```python
from build123d import *

# Parameters (mm, degrees)
SKETCH1_R                = 4.25
EXTRUDE1_DEPTH           = 6
PROCESS_BENDS1_START     = -45.500357344
PROCESS_BENDS1_OUTLINE_W = 30
PROCESS_BENDS1_OUTLINE_H = 6
PROCESS_BENDS1_DEPTH     = 45.500357344
PROCESS_BENDS1_START_2   = -50.267477344
PROCESS_BENDS1_2_DEPTH   = 4.83288
PROCESS_BENDS1_START_3   = -56.267477344
PROCESS_BENDS1_3_DEPTH   = 6
PROCESS_BENDS1_START_4   = -45.434597344
PROCESS_BENDS1_4_DEPTH   = 1.16712
PROCESS_BENDS1_START_5   = -21
PROCESS_BENDS1_5_DEPTH   = 30


with BuildPart() as part:
    # Sketch1 → Extrude1 (new body)
    with BuildSketch(Plane.XY):
        with BuildLine():
            Line((-106.422252789, 9), (-40.637070261, 9))
            ThreePointArc((-40.637070261, 9), (-40.099770652, 8.843391446), (-39.730762474, 8.422618262))
            Line((-39.730762474, 8.422618262), (-38.495606339, 5.773817383))
            ThreePointArc((-38.495606339, 5.773817383), (-34.805524552, 1.566085542), (-29.432528469, 0))
            Line((-29.432528469, 0), (-3, 0))
            ThreePointArc((-3, 0), (-0.878679656, -0.878679656), (0, -3))
            Line((0, -3), (0, -7.904690938))
            ThreePointArc((0, -7.904690938), (-0.540498847, -9.622495956), (-1.967236053, -10.721319886))
            Line((-1.967236053, -10.721319886), (-29.49989713, -20.816628948))
            ThreePointArc((-29.49989713, -20.816628948), (-30.008202711, -20.95380152), (-30.532661077, -21))
            Line((-30.532661077, -21), (-159, -21))
            ThreePointArc((-159, -21), (-161.121320344, -20.121320344), (-162, -18))
            Line((-162, -18), (-162, 12))
            ThreePointArc((-162, 12), (-161.121320344, 14.121320344), (-159, 15))
            Line((-159, 15), (-122.577747211, 15))
            ThreePointArc((-122.577747211, 15), (-122.010424647, 14.94586916), (-121.463575182, 14.785430073))
            Line((-121.463575182, 14.785430073), (-107.536424818, 9.214569927))
            ThreePointArc((-107.536424818, 9.214569927), (-106.989575353, 9.05413084), (-106.422252789, 9))
        make_face()
        with Locations((-67, -6)):
            Circle(SKETCH1_R, mode=Mode.SUBTRACT)
        with Locations((-112, -6)):
            Circle(SKETCH1_R, mode=Mode.SUBTRACT)
    extrude(amount=EXTRUDE1_DEPTH)

    # Process-Bends1: read off the stored shape, not the designer's step
    # Process-Bends1 outline → Process-Bends1 (cut)
    with BuildSketch(Plane.YZ.offset(PROCESS_BENDS1_START)):
        with Locations((-6, 3)):
            Rectangle(PROCESS_BENDS1_OUTLINE_W, PROCESS_BENDS1_OUTLINE_H)
    extrude(amount=PROCESS_BENDS1_DEPTH, mode=Mode.SUBTRACT)

    # Process-Bends1 2 outline → Process-Bends1 2 (add)
    with BuildSketch(Plane.YZ.offset(PROCESS_BENDS1_START_2)):
        with BuildLine():
            Line((5.773817383, -11.236916317), (8.422618262, -10.001760182))
            ThreePointArc((8.422618262, -10.001760182), (8.843391446, -9.632752004), (9, -9.095452395))
            Line((9, -9.095452395), (9, 0))
            Line((9, 0), (-21, 0))
            Line((-21, 0), (-21, -19.199861579))
            ThreePointArc((-21, -19.199861579), (-20.95380152, -19.724319945), (-20.816628948, -20.232625526))
            Line((-20.816628948, -20.232625526), (-10.721319886, -47.765286604))
            ThreePointArc((-10.721319886, -47.765286604), (-9.622495956, -49.192023809), (-7.904690938, -49.732522656))
            Line((-7.904690938, -49.732522656), (-3, -49.732522656))
            ThreePointArc((-3, -49.732522656), (-0.878679656, -48.853843), (0, -46.732522656))
            Line((0, -46.732522656), (0, -20.299994188))
            ThreePointArc((0, -20.299994188), (1.566085542, -14.926998104), (5.773817383, -11.236916317))
        make_face()
    extrude(amount=PROCESS_BENDS1_2_DEPTH)

    # Process-Bends1 3 outline → Process-Bends1 3 (add)
    with BuildSketch(Plane.YZ.offset(PROCESS_BENDS1_START_3)):
        with BuildLine():
            Line((5.773817383, -11.236916317), (8.422618262, -10.001760182))
            ThreePointArc((8.422618262, -10.001760182), (8.843391446, -9.632752004), (9, -9.095452395))
            Line((9, -9.095452395), (9, 0))
            Line((9, 0), (-21, 0))
            Line((-21, 0), (-21, -19.199861579))
            ThreePointArc((-21, -19.199861579), (-20.95380152, -19.724319945), (-20.816628948, -20.232625526))
            Line((-20.816628948, -20.232625526), (-10.721319886, -47.765286604))
            ThreePointArc((-10.721319886, -47.765286604), (-9.622495956, -49.192023809), (-7.904690938, -49.732522656))
            Line((-7.904690938, -49.732522656), (-3, -49.732522656))
            ThreePointArc((-3, -49.732522656), (-0.878679656, -48.853843), (0, -46.732522656))
            Line((0, -46.732522656), (0, -20.299994188))
            ThreePointArc((0, -20.299994188), (1.566085542, -14.926998104), (5.773817383, -11.236916317))
        make_face()
    extrude(amount=PROCESS_BENDS1_3_DEPTH)

    # Process-Bends1 4 outline → Process-Bends1 4 (add)
    with BuildSketch(Plane.YZ.offset(PROCESS_BENDS1_START_4)):
        with BuildLine():
            Line((5.773817383, -11.236916317), (8.422618262, -10.001760182))
            ThreePointArc((8.422618262, -10.001760182), (8.843391446, -9.632752004), (9, -9.095452395))
            Line((9, -9.095452395), (9, 0))
            Line((9, 0), (-21, 0))
            Line((-21, 0), (-21, -19.199861579))
            ThreePointArc((-21, -19.199861579), (-20.95380152, -19.724319945), (-20.816628948, -20.232625526))
            Line((-20.816628948, -20.232625526), (-10.721319886, -47.765286604))
            ThreePointArc((-10.721319886, -47.765286604), (-9.622495956, -49.192023809), (-7.904690938, -49.732522656))
            Line((-7.904690938, -49.732522656), (-3, -49.732522656))
            ThreePointArc((-3, -49.732522656), (-0.878679656, -48.853843), (0, -46.732522656))
            Line((0, -46.732522656), (0, -20.299994188))
            ThreePointArc((0, -20.299994188), (1.566085542, -14.926998104), (5.773817383, -11.236916317))
        make_face()
    extrude(amount=PROCESS_BENDS1_4_DEPTH)

    # Process-Bends1 5 outline → Process-Bends1 5 (cut)
    with BuildSketch(Plane(origin=(0, 0, 0), x_dir=(1, 0, 0), z_dir=(0, 1, 0)).offset(PROCESS_BENDS1_START_5)):
        with BuildLine():
            Line((-50.267477344, 6), (-50.267477344, 49.732522656))
            Line((-50.267477344, 49.732522656), (-56.267477344, 49.732522656))
            Line((-56.267477344, 49.732522656), (-56.267477344, 0))
            ThreePointArc((-56.267477344, 0), (-52.024836657, 1.757359313), (-50.267477344, 6))
        make_face()
        with BuildLine():
            Line((-44.267477344, 0), (-44.267477344, 6))
            ThreePointArc((-44.267477344, 6), (-47.78219597, -2.485281374), (-56.267477344, -6))
            Line((-56.267477344, -6), (-45.500357344, -6))
            Line((-45.500357344, -6), (-45.500357344, 0))
            Line((-45.500357344, 0), (-44.267477344, 0))
        make_face()
    extrude(amount=PROCESS_BENDS1_5_DEPTH, mode=Mode.SUBTRACT)


solid = part.part
```
The model under review builds one solid part; all positions refer to its coordinate system, in mm. A direction names the side the tool comes from. Give positions to 0.01 mm unless a question says otherwise; leave off trailing zeros. Write each loop counter-clockwise with the first axis right and the second up, starting at its lowest first coordinate (ties: lowest second). Pieces come first, ordered by that corner, then holes. Notation, with made-up numbers: M 77,-19.5 L 109,-19.5 A31 ccw 109,17.5 Z; hole C 13.5,12.25 d5. An arc over 180 degrees is marked long. Write each question's results on one line, items separated by ' | '. Start each with the question number.
1. We need section C-C (x = -112). Write out the cut boundary in (y, z).
2. For probe 1 along Y at (x, z) = (-67, 3.3); probe 2 along X at (y, z) = (-13.5, -13.5); probe 3 along Z at (x, y) = (-81, -13), list the stretches that pass through material, from the lowest coordinate up. Write a range as [from, to].
3. Insertion check: pin 1 Ø12 at (x, z) = (-80.5, -1) entering from +Y; pin 2 Ø5 at (x, y) = (-70, 4) entering from -Z; pin 3 Ø5 at (x, z) = (-48, -31.5) entering from +Y. Each pin has a flat end and moves straight along its axis. Give the tip position at first contact, or say it passes through.
4. For faces 5 (the flat face through (-76, 9, 2)), 6 (the flat face through (-47, 0, -34)), 7 (the flat face through (-108, -3, 0)), list the 3-axis set-ups (+Z, -Z, +X, -X, +Y, -Y) from which the entire face can be reached by the end or side of a thin tool; tool diameter is ignored.
5. Mouldability with a two-part tool opening along Y and no side actions: class faces 1 (the flat face through (-141, 15, 3)), 2 (the cylindrical face through (-62.946, -4.723, 2.958)), 3 (the cylindrical face through (-116.246, -5.813, 2.958)), 4 (the flat face through (-93, -21, 2)) as released by +Y, released by -Y, zero draft, split by the parting line, or undercut.
6. We need section A-A (x = -67). Write out the cut boundary in (y, z), and give its area (3 significant figures).
7. We need section D-D (z = -17.5). Write out the cut boundary in (x, y).
8. We need section B-B (y = -6). Write out the cut boundary in (x, z).
Results found:
1) outline: M -21,0 L -10.25,0 L -10.25,6 L -21,6 Z; M -1.75,0 L 11,0 L 11,6 L -1.75,6 Z
2) probe 1: y = [-21, -10.25], [-1.75, 9] | probe 2: x = [-50.27, -44.27] | probe 3: z = [0, 6]
3) pin 1: stops at y = 9 | pin 2: stops at z = 0 | pin 3: stops at y = 0
4) face 5: +Z, -Z, +X, +Y | face 6: -Z, +X, -X, +Y | face 7: -Z, -X, +Y, -Y
5) face 1: released by +Y | face 2: undercut | face 3: undercut | face 4: released by -Y
6) outline: M -21,0 L -10.25,0 L -10.25,6 L -21,6 Z; M -1.75,0 L 9,0 L 9,6 L -1.75,6 Z | area: 129 mm^2
7) outline: M -50.27,-21 L -44.27,-21 L -44.27,0.4 L -50.27,0.4 Z
8) outline: M -162,0 L -116.25,0 L -116.25,6 L -162,6 Z; M -107.75,0 L -71.25,0 L -71.25,6 L -107.75,6 Z; M -62.75,0 L -56.27,0 A6 cw -50.27,-6 L -50.27,-49.73 L -44.27,-49.73 L -44.27,-6 A12 ccw -56.27,6 L -62.75,6 Z
